The listing builds one solid part. Answer for the finished solid, in the listing's coordinates (mm). Face numbers are marked on the shaded views. A direction names the side the tool comes from. Coordinates: 2 decimals unless noted, no trailing zeros. Order: outer loops, then holes, each group sorted by start corner. A loop starts at its lowest first (then second) coordinate and runs counter-clockwise, first axis right, second up. Notation, with made-up numbers: (31.25, -38) -> (88.25, -38) arc R7 cw to (88.25, -26) -> close; hole circle Ø1 at (77.25, 34.5). An arc over 180 degrees is marked (long way). Put each result on its own line as item: value. Start each with the question number.
```python
from build123d import *

# Parameters (mm, degrees)
SKETCH_1_R               = 25.5
SKETCH_1_R_2             = 2.5
EXTRUDE_1_DEPTH          = 8
SKETCH_2_R               = 7.5
SKETCH_2_R_2             = 2.5
EXTRUDE_2_DEPTH          = 8
CUT_EXTRUDE_2_DEPTH      = 10
CUT_EXTRUDE_2_DEPTH_BACK = 10
SKETCH_4_R               = 1.25
SKETCH_6_R               = 2


with BuildPart() as part:
    # Sketch 1 → Extrude 1 (new body)
    with BuildSketch(Plane.XY):
        Circle(SKETCH_1_R)
        Circle(SKETCH_1_R_2, mode=Mode.SUBTRACT)
    extrude(amount=EXTRUDE_1_DEPTH)

    # Sketch 2 → Extrude 2 (add)
    with BuildSketch(Plane.XY.offset(8)):
        Circle(SKETCH_2_R)
        Circle(SKETCH_2_R_2, mode=Mode.SUBTRACT)
    extrude(amount=EXTRUDE_2_DEPTH)

    # Sketch 4 → Cut-Extrude 2 (cut, two sides: drawn at the far end of the back side and taken through both)
    with BuildSketch(Plane(origin=(0, 0, 0), x_dir=(1, 0, 0), z_dir=(0, 1, 0)).offset(-CUT_EXTRUDE_2_DEPTH_BACK)):
        with Locations(Location((0, -12, 0), (0, 0, 90))):
            Circle(SKETCH_4_R)
    extrude(amount=CUT_EXTRUDE_2_DEPTH + CUT_EXTRUDE_2_DEPTH_BACK, mode=Mode.SUBTRACT)

    # Sketch 5 → Cut-Revolve 1 (revolve, cut)
    with BuildSketch(Plane(origin=(0, 0, 0), x_dir=(0, 0, -1), z_dir=(1, 0, 0)), mode=Mode.PRIVATE) as cut_revolve_1_sk:
        with BuildLine():
            Line((-6, 25.5), (-2, 25.5))
            ThreePointArc((-2, 25.5), (-4, 23.5), (-6, 25.5))
        make_face()
    revolve(cut_revolve_1_sk.sketch.rotate(Axis((0, 0, 0), (0, 0, 1)), 90), axis=Axis((0, 0, 0), (0, 0, 1)), mode=Mode.SUBTRACT)

    # Sketch 6 → Revolve 1 (revolve)
    with BuildSketch(Plane(origin=(0, 0, 0), x_dir=(0, 0, -1), z_dir=(1, 0, 0)), mode=Mode.PRIVATE) as revolve_1_sk:
        with Locations((-4, 25.5)):
            Circle(SKETCH_6_R)
    revolve(revolve_1_sk.sketch.rotate(Axis((0, 0, 0), (0, 0, 1)), 90), axis=Axis((0, 0, 0), (0, 0, 1)))


solid = part.part
```
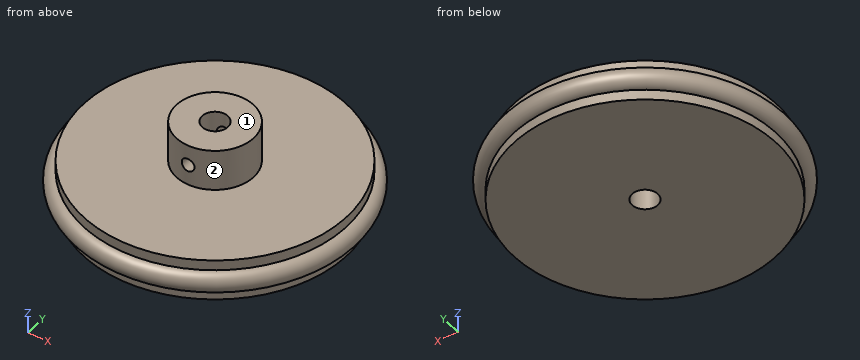
(1) Find the intervals of material crossed by L1, parallel to Y at x = 0, z = 7.5; L2, parallel to Z at x = -5, y = -24; L3, parallel to X at y = 3.4, z = 12, in increasing order.
(2) A tool of negligible diameter and unlimited length cuts with its end or side. For the marked faces 1 and 2, from which of +Z, -Z, +X, -X, +Y, -Y can it reach the whole face along a straight path? Write none if from no direction.
(3) The part is cut by section A-A on y = 0. Determine the outline of the cut face in (x, z).
(4) Each of these flat-tipped pins is pushed along its axis until it touches: P1, Ø1.5, axis at x = 0, z = 12, coming from the +Y side; P2, Ø1, axis at x = -9, y = 4, coming from the +Z side. Where does it stop, or does it pass through?
(5) The part is cut by section D-D on z = 2.75. Determine the outline of the cut face in (x, y).
(6) The part is cut by section B-B on x = 0. Determine the outline of the cut face in (y, z).
(7) The part is cut by section C-C on z = 12. Determine the outline of the cut face in (x, y).
Worked out:
1. L1: -25.5 to -2.5, 2.5 to 25.5
1. L2: 0 to 8
1. L3: -6.69 to -1.25, 1.25 to 6.69
2. face 1: +Z, +X, -X, +Y, -Y
2. face 2: +Z
3. outline: (-25.5, 0) -> (-2.5, 0) -> (-2.5, 16) -> (-7.5, 16) -> (-7.5, 8) -> (-25.5, 8) -> (-25.5, 6) arc R2 ccw to (-25.5, 2) -> close; (2.5, 0) -> (25.5, 0) -> (25.5, 2) arc R2 ccw to (25.5, 6) -> (25.5, 8) -> (7.5, 8) -> (7.5, 16) -> (2.5, 16) -> close
4. P1: through
4. P2: z = 8
5. outline: circle Ø54.12 at (0, 0); hole circle Ø5 at (0, 0)
6. outline: (-25.5, 0) -> (-2.5, 0) -> (-2.5, 10.75) -> (-7.5, 10.75) -> (-7.5, 8) -> (-25.5, 8) -> (-25.5, 6) arc R2 ccw to (-25.5, 2) -> close; (-7.5, 13.25) -> (-2.5, 13.25) -> (-2.5, 16) -> (-7.5, 16) -> close; (2.5, 0) -> (25.5, 0) -> (25.5, 2) arc R2 ccw to (25.5, 6) -> (25.5, 8) -> (7.5, 8) -> (7.5, 10.75) -> (2.5, 10.75) -> close; (2.5, 13.25) -> (7.5, 13.25) -> (7.5, 16) -> (2.5, 16) -> close
7. outline: (-1.25, -7.4) -> (-1.25, -2.17) arc R2.5 cw to (-1.25, 2.17) -> (-1.25, 7.4) arc R7.5 ccw to start; (1.25, -7.4) arc R7.5 ccw to (1.25, 7.4) -> (1.25, 2.17) arc R2.5 cw to (1.25, -2.17) -> close
